Work out the finished part from the listing and answer in its coordinate system (mm). Round coordinates to 2 decimals unless told otherwise and drop trailing zeros. Write each loop counter-clockwise with the first axis right and the second up, starting at its lowest first coordinate (ties: lowest second). Pieces come first, ordered by that corner, then holes. Notation, with made-up numbers: M 84,-5.5 L 110,-5.5 A37 cw 110,30.5 Z; hole C 39,16 d9. An arc over 180 degrees is marked long. One line per item, written item: value. Start each with the question number.
Q1. Find section C-C (z = 1.65). Count the separate pieces of the cut face and the enclosed holes in it, and give its area (3 significant figures).
Q2. Find section B-B (y = 27). Write down the section's boundary in (x, z).
Q3. Find section A-A (x = 72). Write down the section's boundary in (y, z).
Q4. Consider probe 1 along X at (y, z) = (25, 3.55); probe 2 along X at (y, z) = (35, 0.9); probe 3 along Y at (x, z) = (-51.5, 2.1). Determine where each line is inside the solid, lowest interval first.
Q5. The mould has two halves that part along X. Classify faces 1 (the flat face through (111, 33.115, 2)), 2 (the flat face through (19, 40.115, 2)): released by +X, released by -X, zero draft, split by the parting line, or undercut.
from build123d import *

# Parameters (mm, degrees)
SKETCH2_W           = 200
SKETCH2_H           = 32
BOSS_EXTRUDE1_DEPTH = 4
SKETCH3_W           = 43
SKETCH3_H           = 21.6
SKETCH3_W_2         = 6
SKETCH3_H_2         = 5.15
SKETCH3_W_3         = 5
SKETCH3_W_4         = 4
SKETCH3_H_3         = 18
SKETCH3_H_4         = 5.2
CUT_EXTRUDE1_DEPTH  = 4


with BuildPart() as part:
    # Sketch2 → Boss-Extrude1 (new body)
    with BuildSketch(Plane.XY):
        with Locations((20.66568498, 24.11539075)):
            Rectangle(SKETCH2_W, SKETCH2_H)
    extrude(amount=BOSS_EXTRUDE1_DEPTH)

    # Sketch3 → Cut-Extrude1 (cut)
    with BuildSketch(Plane.XY.offset(4)):
        with Locations((-20.83431502, 24.11539075)):
            Rectangle(SKETCH3_W, SKETCH3_H)
        with Locations((62.16568498, 24.11539075)):
            Rectangle(SKETCH3_W, SKETCH3_H)
        with Locations((31.66568498, 32.69039075)):
            Rectangle(SKETCH3_W_2, SKETCH3_H_2)
        with Locations((-51.33431502, 32.69039075)):
            Rectangle(SKETCH3_W_2, SKETCH3_H_2)
        with Locations((-50.83431502, 15.54039075)):
            Rectangle(SKETCH3_W_3, SKETCH3_H_2)
        with Locations((9.66568498, 32.69039075)):
            Rectangle(SKETCH3_W_2, SKETCH3_H_2)
        with Locations((9.66568498, 15.54039075)):
            Rectangle(SKETCH3_W_2, SKETCH3_H_2)
        with Locations((-69.33431502, 24.11539075)):
            Rectangle(SKETCH3_W_4, SKETCH3_H_3)
        with Locations((31.66568498, 15.54039075)):
            Rectangle(SKETCH3_W_2, SKETCH3_H_2)
        with Locations((92.16568498, 32.71539075)):
            Rectangle(SKETCH3_W_3, SKETCH3_H_4)
        with Locations((92.66568498, 15.54039075)):
            Rectangle(SKETCH3_W_2, SKETCH3_H_2)
        with Locations((110.66568498, 24.11539075)):
            Rectangle(SKETCH3_W_4, SKETCH3_H_3)
    extrude(amount=-CUT_EXTRUDE1_DEPTH, mode=Mode.SUBTRACT)


solid = part.part
The answers:
1. separate pieces: 1
1. enclosed holes: 12
1. area: 4,160 mm2
2. outline: M -79.33,0 L -71.33,0 L -71.33,4 L -79.33,4 Z; M -67.33,0 L -42.33,0 L -42.33,4 L -67.33,4 Z; M 0.67,0 L 40.67,0 L 40.67,4 L 0.67,4 Z; M 83.67,0 L 108.67,0 L 108.67,4 L 83.67,4 Z; M 112.67,0 L 120.67,0 L 120.67,4 L 112.67,4 Z
3. outline: M 8.12,0 L 13.32,0 L 13.32,4 L 8.12,4 Z; M 34.92,0 L 40.12,0 L 40.12,4 L 34.92,4 Z
4. probe 1: -79.33 to -71.33, -67.33 to -42.33, 0.67 to 40.67, 83.67 to 108.67, 112.67 to 120.67
4. probe 2: -79.33 to -54.33, -48.33 to 6.67, 12.67 to 28.67, 34.67 to 89.67, 94.67 to 120.67
4. probe 3: 8.12 to 12.97, 18.12 to 30.12, 35.27 to 40.12
5. face 1: undercut
5. face 2: zero draft
